Can you work these out from the model? Positions are in its coordinate system, mm. Face numbers are marked on the shaded views. A direction names the side the tool comes from. Round coordinates to 2 decimals unless told otherwise and drop trailing zeros. Order: outer loops, then holes, each group sorted by start corner. A loop starts at its lowest first (then second) coordinate and runs counter-clockwise, first axis right, second up. Notation, with made-up numbers: (74.25, 62) -> (129.25, 62) arc R13 ccw to (129.25, 86) -> close; hole circle Ø1 at (56, 82.5). An arc over 180 degrees is marked (long way). One line per item, written item: value.
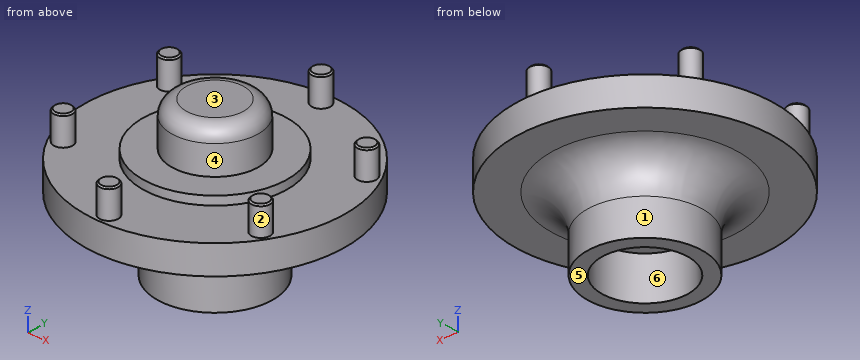
```python
from build123d import *

# Parameters (mm, degrees)
SKETCH7_R           = 6.5
BOSS_EXTRUDE2_DEPTH = 20
FILLET2_R           = 25
FILLET2_2_R         = 10
CHAMFER1_SIZE       = 1


with BuildPart() as part:
    # Sketch6 → Revolve2 (revolve)
    with BuildSketch(Plane(origin=(0, 0, -433528.712964682), x_dir=(-1, 0, 0), z_dir=(0, -1, 0))):
        Polygon((-30, -433528.712964682), (0, -433528.712964682), (0, -433452.712964682), (-30, -433452.712964682), (-30, -433422.712964682), (-40, -433422.712964682), (-40, -433472.712964682), (-90, -433472.712964682), (-90, -433492.712964682), (-50, -433492.712964682), (-50, -433498.712964682), (-30, -433498.712964682), align=None)
    revolve(axis=Axis((0, 0, 0), (0, 0, -1)))

    # Sketch7 → Boss-Extrude2 (add)
    with BuildSketch(Plane(origin=(0, 0, -36), x_dir=(-1, 0, 0), z_dir=(0, 0, 1))):
        with Locations((70.581070408, 40.75)):
            Circle(SKETCH7_R)
        with Locations((0, 81.5)):
            Circle(SKETCH7_R)
        with Locations((70.581070408, -40.75)):
            Circle(SKETCH7_R)
        with Locations((0, -81.5)):
            Circle(SKETCH7_R)
        with Locations((-70.581070408, -40.75)):
            Circle(SKETCH7_R)
        with Locations((-70.581070408, 40.75)):
            Circle(SKETCH7_R)
    extrude(amount=BOSS_EXTRUDE2_DEPTH)

    # Fillet2
    fillet2_edges = [part.edges().sort_by_distance(p)[0] for p in [
        (-40, 0, -56),
    ]]
    fillet(fillet2_edges, radius=FILLET2_R)

    # Fillet2 2
    fillet2_2_edges = [part.edges().sort_by_distance(p)[0] for p in [
        (-30, 0, 0),
    ]]
    fillet(fillet2_2_edges, radius=FILLET2_2_R)

    # Chamfer1
    chamfer1_edges = [part.edges().sort_by_distance(p)[0] for p in [
        (-64.081070408, -40.75, -16),
        (6.5, -81.5, -16),
        (-64.081070408, 40.75, -16),
        (6.5, 81.5, -16),
        (77.081070408, 40.75, -16),
        (77.081070408, -40.75, -16),
    ]]
    chamfer(chamfer1_edges, length=CHAMFER1_SIZE)


solid = part.part
```
Q1. Will these pins go through, and if not, where does the flat tip stop? pin 1 Ø3.5 at (x, y) = (71.5, 39) entering from +Z; pin 2 Ø12 at (x, y) = (49, 35.5) entering from +Z; pin 3 Ø6 at (x, z) = (-49.5, -43.5) entering from -Y.
Answers below:
pin 1: z = -16
pin 2: z = -36
pin 3: y = -77.06
Q2. On a 3-axis mill with a long thin cutter (end or side, diameter ignored), from which of +Z, -Z, +X, -X, +Y, -Y can I reach the whole of each face in a straight line? I mean the marked faces 4, 5 and 6. Say none if no direction works.
Answers below:
face 4: +Z
face 5: -Z, +X, -X, +Y, -Y
face 6: -Z
Q3. I want a section at C-C on z = -49.5. List the corners of the cut face in (x, y) for me, plus the area to 3 significant figures.
Answers below:
outline: circle Ø180 at (0, 0)
area: 25,400 mm^2
Q4. I want a section at D-D on y = -81.5. List the corners of the cut face in (x, z) for me.
Answers below:
outline: (-38.18, -56) -> (38.18, -56) -> (38.18, -36) -> (6.5, -36) -> (6.5, -17) -> (5.5, -16) -> (-5.5, -16) -> (-6.5, -17) -> (-6.5, -36) -> (-38.18, -36) -> close
Q5. I want a section at A-A on z = -26. List the corners of the cut face in (x, y) for me, plus the area to 3 significant figures.
Answers below:
outline: circle Ø13 at (-70.58, -40.75); circle Ø13 at (-70.58, 40.75); circle Ø60 at (0, 0); circle Ø13 at (0, -81.5); circle Ø13 at (0, 81.5); circle Ø13 at (70.58, -40.75); circle Ø13 at (70.58, 40.75)
area: 3,620 mm^2
Q6. Please list where these lines run through material, in increasing order: line 1 along Y through (x, z) = (0, -85.5); line 2 along Z through (x, y) = (25.5, 74).
Answers below:
line 1: -40 to -30, 30 to 40
line 2: -56 to -36
Q7. I want a section at B-B on y = 0. List the corners of the cut face in (x, z) for me.
Answers below:
outline: (-90, -56) -> (-65, -56) arc R25 cw to (-40, -81) -> (-40, -106) -> (-30, -106) -> (-30, -76) -> (30, -76) -> (30, -106) -> (40, -106) -> (40, -81) arc R25 cw to (65, -56) -> (90, -56) -> (90, -36) -> (50, -36) -> (50, -30) -> (30, -30) -> (30, -10) arc R10 ccw to (20, 0) -> (-20, 0) arc R10 ccw to (-30, -10) -> (-30, -30) -> (-50, -30) -> (-50, -36) -> (-90, -36) -> close
Q8. We'd pull the mould along Y, two halves only. Please class the marked faces 1, 2 and 3: released by +Y, released by -Y, zero draft, split by the parting line, or undercut.
Answers below:
face 1: split by the parting line
face 2: undercut
face 3: zero draft
